from build123d import *

# Parameters (mm, degrees)
SKETCH1_W           = 42
SKETCH1_H           = 42
BOSS_EXTRUDE1_DEPTH = 25
SKETCH2_R           = 3
BOSS_EXTRUDE2_DEPTH = 11
CUT_EXTRUDE1_DEPTH  = 42
SKETCH4_R           = 1.5
CUT_EXTRUDE2_DEPTH  = 100
CHAMFER2_SIZE       = 5


with BuildPart() as part:
    # Sketch1 → Boss-Extrude1 (new body)
    with BuildSketch(Plane(origin=(0, 0, 0), x_dir=(0, 0, -1), z_dir=(1, 0, 0))):
        with Locations((21, 21)):
            Rectangle(SKETCH1_W, SKETCH1_H)
    extrude(amount=BOSS_EXTRUDE1_DEPTH)

    # Sketch2 → Boss-Extrude2 (add)
    with BuildSketch(Plane.XZ):
        with Locations(Location((18, -17, 0), (0, 0, 90))):
            Circle(SKETCH2_R)
    extrude(amount=BOSS_EXTRUDE2_DEPTH)

    # Sketch3 → Cut-Extrude1 (cut)
    with BuildSketch(Plane(origin=(25, 0, 0), x_dir=(0, 0, -1), z_dir=(1, 0, 0))):
        with BuildLine():
            ThreePointArc((8, 36), (4.585786438, 37.414213562), (6, 34))
            Line((6, 34), (6, 36))
            Line((6, 36), (8, 36))
        make_face()
        with BuildLine():
            Line((6, 36), (6, 34))
            ThreePointArc((6, 34), (7.414213562, 34.585786438), (8, 36))
            Line((8, 36), (6, 36))
        make_face()
        with BuildLine():
            ThreePointArc((34, 36), (34.585786438, 34.585786438), (36, 34))
            Line((36, 34), (36, 36))
            Line((36, 36), (34, 36))
        make_face()
        with BuildLine():
            Line((36, 36), (36, 34))
            ThreePointArc((36, 34), (37.414213562, 34.585786438), (38, 36))
            ThreePointArc((38, 36), (36, 38), (34, 36))
            Line((34, 36), (36, 36))
        make_face()
        with BuildLine():
            Line((6, 8), (6, 6))
            Line((6, 6), (8, 6))
            ThreePointArc((8, 6), (7.414213562, 7.414213562), (6, 8))
        make_face()
        with BuildLine():
            Line((8, 6), (6, 6))
            Line((6, 6), (6, 8))
            ThreePointArc((6, 8), (4.585786438, 4.585786438), (8, 6))
        make_face()
        with BuildLine():
            ThreePointArc((36, 8), (34.585786438, 7.414213562), (34, 6))
            Line((34, 6), (36, 6))
            Line((36, 6), (36, 8))
        make_face()
        with BuildLine():
            Line((36, 6), (34, 6))
            ThreePointArc((34, 6), (36, 4), (38, 6))
            ThreePointArc((38, 6), (37.414213562, 7.414213562), (36, 8))
            Line((36, 8), (36, 6))
        make_face()
    extrude(amount=-CUT_EXTRUDE1_DEPTH, mode=Mode.SUBTRACT)

    # Sketch4 → Cut-Extrude2 (cut)
    with BuildSketch(Plane.XZ.offset(11)):
        with Locations(Location((18, -17, 0), (0, 0, 270))):
            Circle(SKETCH4_R)
    extrude(amount=-CUT_EXTRUDE2_DEPTH, mode=Mode.SUBTRACT)

    # Chamfer2
    chamfer2_edges = [part.edges().sort_by_distance(p)[0] for p in [
        (12.5, 42, 0),
        (12.5, 42, -42),
        (12.5, 0, -42),
        (12.5, 0, 0),
    ]]
    chamfer(chamfer2_edges, length=CHAMFER2_SIZE)


solid = part.part
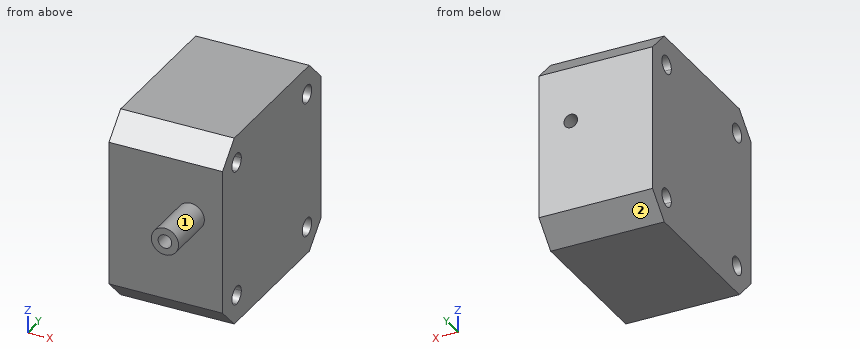
Verification items for the finished model (mm, model axes). Face numbers are marked on the shaded views. A direction names the side the tool comes from. Give positions to 0.01 mm unless a question says otherwise; leave off trailing zeros. Loops run counter-clockwise (first coordinate to the right, second up) from the corner with the lowest first, then second, coordinate; pieces in that order, holes last.
1. Tool access check on the marked faces 1 and 2. Record the directions out of +Z, -Z, +X, -X, +Y, -Y that give a thin tool (end or side, any length) a straight path to the whole face; none if there is none.
Derived:
face 1: -Y
face 2: -Z, +X, -X, +Y
2. Material ranges on probe 1 along Y at (x, z) = (20.25, -6); probe 2 along Z at (x, y) = (10.5, 36); probe 3 along Y at (x, z) = (12.5, -35), recorded low to high.
Derived:
probe 1: y = 0 to 4, 8 to 34, 38 to 42
probe 2: z = -42 to -38, -34 to -8, -4 to 0
probe 3: y = 0 to 4.27, 7.73 to 34.27, 37.73 to 42
3. Cross-section at C-C on x = 22.25. Record the cut outline in (y, z), and give its area (3 significant figures).
Derived:
outline: (0, -37) - (5, -42) - (37, -42) - (42, -37) - (42, -5) - (37, 0) - (5, 0) - (0, -5) - close; hole circle Ø4 at (6, -36); hole circle Ø4 at (6, -6); hole circle Ø4 at (36, -36); hole circle Ø4 at (36, -6)
area: 1,660 mm2
4. Cross-section at A-A on x = 18. Record the cut outline in (y, z).
Derived:
outline: (-11, -20) - (0, -20) - (0, -37) - (5, -42) - (37, -42) - (42, -37) - (42, -18.5) - (-11, -18.5) - close; (-11, -15.5) - (42, -15.5) - (42, -5) - (37, 0) - (5, 0) - (0, -5) - (0, -14) - (-11, -14) - close; hole circle Ø4 at (6, -36); hole circle Ø4 at (6, -6); hole circle Ø4 at (36, -36); hole circle Ø4 at (36, -6)
5. Go/stop test with flat-tipped pins: P1, Ø3, axis at y = 6, z = -6, coming from the -X side; P2, Ø12.5, axis at x = 8, z = -24.5, coming from the -Y side. Record where each tip stops, or that it passes through.
Derived:
P1: passes through
P2: stops at y = 0
6. Cross-section at D-D on z = -12.5. Record the cut outline in (x, y), and give its area (3 significant figures).
Derived:
outline: (0, 0) - (25, 0) - (25, 42) - (0, 42) - close
area: 1,050 mm2
7. Cross-section at B-B on y = 1.5. Record the cut outline in (x, z).
Derived:
outline: (0, -38.5) - (25, -38.5) - (25, -3.5) - (0, -3.5) - close; hole circle Ø3 at (18, -17)
